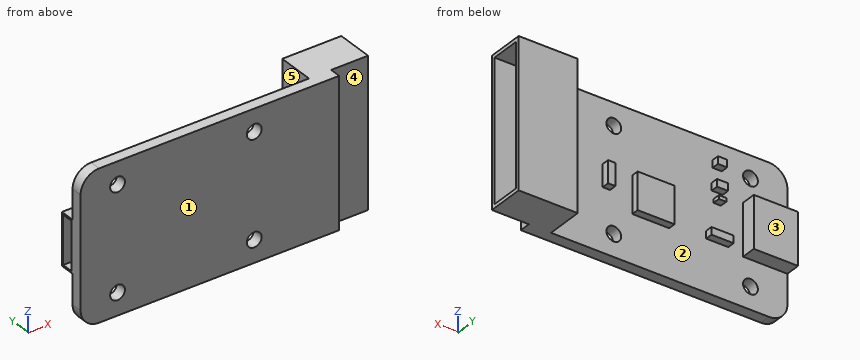
```python
from build123d import *

# Parameters (mm, degrees)
SKETCH1_W           = 35
SKETCH1_H           = 20
BOSS_EXTRUDE1_DEPTH = 1.5
FILLET1_R           = 2.5
SKETCH2_R           = 1
CUT_EXTRUDE1_DEPTH  = 1.5
SKETCH3_W           = 6
SKETCH3_H           = 7
BOSS_EXTRUDE2_DEPTH = 2
SKETCH4_W           = 6.5
SKETCH4_H           = 1.5
CUT_EXTRUDE2_DEPTH  = 5.5
SKETCH5_W           = 8
SKETCH5_H           = 20
BOSS_EXTRUDE3_DEPTH = 5
SKETCH6_W           = 19
SKETCH6_H           = 4
CUT_EXTRUDE3_DEPTH  = 7
SKETCH7_W           = 5
SKETCH7_H           = 5
BOSS_EXTRUDE4_DEPTH = 1
SKETCH8_W           = 1.25
SKETCH8_H           = 1
SKETCH8_W_2         = 1.5
SKETCH8_W_3         = 1
SKETCH8_H_2         = 0.5
SKETCH8_W_4         = 3
SKETCH8_H_3         = 3
BOSS_EXTRUDE5_DEPTH = 1


with BuildPart() as part:
    # Sketch1 → Boss-Extrude1 (new body)
    with BuildSketch(Plane(origin=(0, 0, 0), x_dir=(1, 0, 0), z_dir=(0, 1, 0))):
        Rectangle(SKETCH1_W, SKETCH1_H)
    extrude(amount=BOSS_EXTRUDE1_DEPTH)

    # Fillet1
    fillet1_edges = [part.edges().sort_by_distance(p)[0] for p in [
        (-17.5, 0.75, 10),
        (-17.5, 0.75, -10),
    ]]
    fillet(fillet1_edges, radius=FILLET1_R)

    # Sketch2 → Cut-Extrude1 (cut)
    with BuildSketch(Plane(origin=(0, 1.5, 0), x_dir=(1, 0, 0), z_dir=(0, 1, 0))):
        with Locations((-12.5, 7)):
            Circle(SKETCH2_R)
        with Locations((6, 7)):
            Circle(SKETCH2_R)
        with Locations((6, -7)):
            Circle(SKETCH2_R)
        with Locations((-12.5, -7)):
            Circle(SKETCH2_R)
    extrude(amount=-CUT_EXTRUDE1_DEPTH, mode=Mode.SUBTRACT)

    # Sketch3 → Boss-Extrude2 (add)
    with BuildSketch(Plane(origin=(0, 1.5, 0), x_dir=(1, 0, 0), z_dir=(0, 1, 0))):
        with Locations((-14.5, 0)):
            Rectangle(SKETCH3_W, SKETCH3_H)
    extrude(amount=BOSS_EXTRUDE2_DEPTH)

    # Sketch4 → Cut-Extrude2 (cut)
    with BuildSketch(Plane.ZY.offset(17.5)):
        with Locations((0, 2.5)):
            Rectangle(SKETCH4_W, SKETCH4_H)
    extrude(amount=-CUT_EXTRUDE2_DEPTH, mode=Mode.SUBTRACT)

    # Sketch5 → Boss-Extrude3 (add)
    with BuildSketch(Plane(origin=(0, 1.5, 0), x_dir=(1, 0, 0), z_dir=(0, 1, 0))):
        with Locations((18.5, 0)):
            Rectangle(SKETCH5_W, SKETCH5_H)
    extrude(amount=BOSS_EXTRUDE3_DEPTH)

    # Sketch6 → Cut-Extrude3 (cut)
    with BuildSketch(Plane(origin=(22.5, 0, 0), x_dir=(0, 0, -1), z_dir=(1, 0, 0))):
        with Locations((0, 4)):
            Rectangle(SKETCH6_W, SKETCH6_H)
    extrude(amount=-CUT_EXTRUDE3_DEPTH, mode=Mode.SUBTRACT)

    # Sketch7 → Boss-Extrude4 (add)
    with BuildSketch(Plane(origin=(0, 1.5, 0), x_dir=(1, 0, 0), z_dir=(0, 1, 0))):
        with Locations((1, 1)):
            Rectangle(SKETCH7_W, SKETCH7_H)
    extrude(amount=BOSS_EXTRUDE4_DEPTH)

    # Sketch8 → Boss-Extrude5 (add)
    with BuildSketch(Plane(origin=(0, 1.5, 0), x_dir=(1, 0, 0), z_dir=(0, 1, 0))):
        with Locations((-8, -7)):
            Rectangle(SKETCH8_W, SKETCH8_H)
        with Locations((-8, -4)):
            Rectangle(SKETCH8_W_2, SKETCH8_H)
        with Locations((-8, -2.25)):
            Rectangle(SKETCH8_W_3, SKETCH8_H_2)
        with Locations((-8, 2.5)):
            Rectangle(SKETCH8_W_4, SKETCH8_H)
        with Locations((7, 0)):
            Rectangle(SKETCH8_W_3, SKETCH8_H_3)
    extrude(amount=BOSS_EXTRUDE5_DEPTH)


solid = part.part
```
Could you check a few things on this model? Use its own coordinates, in mm. Face numbers are marked on the shaded views. A direction names the side the tool comes from. Coordinates: 2 decimals unless noted, no trailing zeros. Loops run counter-clockwise (first coordinate to the right, second up) from the corner with the lowest first, then second, coordinate; pieces in that order, holes last.
1) Thinking about a two-plate mould opening in X: for the marked faces 1 and 2, which applies, released by +X, released by -X, zero draft, split by the parting line, or undercut?
Reported:
face 1: zero draft
face 2: undercut
2) Imagine slicing it at D-D (x = 6). List the corners of the cut face in (y, z) for me, and give its area (3 significant figures).
Reported:
outline: (0, -10) - (1.5, -10) - (1.5, -8) - (0, -8) - close; (0, -6) - (1.5, -6) - (1.5, 6) - (0, 6) - close; (0, 8) - (1.5, 8) - (1.5, 10) - (0, 10) - close
area: 24.0 mm2
3) Which directions (+Z, -Z, +X, -X, +Y, -Y) give clear straight access to the entire face, cutting with the end or side of a thin tool? Please do the marked faces 3, 4 and 5.
Reported:
face 3: +Z, -Z, -X, +Y
face 4: +Z, -Z, +X, -Y
face 5: +Z, -Z, +Y
4) Will these pins go through, and if not, where does the flat tip stop? pin 1 Ø10 at (x, z) = (7, 3) entering from +Y; pin 2 Ø0.5 at (x, y) = (-7.5, 2) entering from -Z; pin 3 Ø0.6 at (y, z) = (2.5, 0.5) entering from +X.
Reported:
pin 1: stops at y = 2.5
pin 2: stops at z = -3
pin 3: stops at x = 15.5
5) Imagine slicing it at A-A (z = 7). List the corners of the cut face in (x, y) for me (3 decimals).
Reported:
outline: (-17.5, 0) - (-13.5, 0) - (-13.5, 1.5) - (-17.5, 1.5) - close; (-11.5, 0) - (5, 0) - (5, 1.5) - (-7.375, 1.5) - (-7.375, 2.5) - (-8.625, 2.5) - (-8.625, 1.5) - (-11.5, 1.5) - close; (7, 0) - (17.5, 0) - (17.5, 1.5) - (22.5, 1.5) - (22.5, 2) - (15.5, 2) - (15.5, 6) - (22.5, 6) - (22.5, 6.5) - (14.5, 6.5) - (14.5, 1.5) - (7, 1.5) - close
6) Imagine slicing it at B-B (x = -12.5). List the corners of the cut face in (y, z) for me.
Reported:
outline: (0, -10) - (1.5, -10) - (1.5, -8) - (0, -8) - close; (0, -6) - (1.5, -6) - (1.5, -3.5) - (3.5, -3.5) - (3.5, 3.5) - (1.5, 3.5) - (1.5, 6) - (0, 6) - close; (0, 8) - (1.5, 8) - (1.5, 10) - (0, 10) - close; hole (1.75, -3.25) - (3.25, -3.25) - (3.25, 3.25) - (1.75, 3.25) - close
7) Imagine slicing it at C-C (y = 5). List the corners of the cut face in (x, z) for me.
Reported:
outline: (14.5, -10) - (22.5, -10) - (22.5, -9.5) - (15.5, -9.5) - (15.5, 9.5) - (22.5, 9.5) - (22.5, 10) - (14.5, 10) - close
8) Please list where these lines run through material, in increasing order: line 1 along X through (y, z) = (0.45, 7); line 2 along Z through (x, y) = (-12.5, 0.85); line 3 along Y through (x, z) = (-7, -6.5).
Reported:
line 1: x = -17.5 to -13.5, -11.5 to 5, 7 to 17.5
line 2: z = -10 to -8, -6 to 6, 8 to 10
line 3: y = 0 to 1.5
